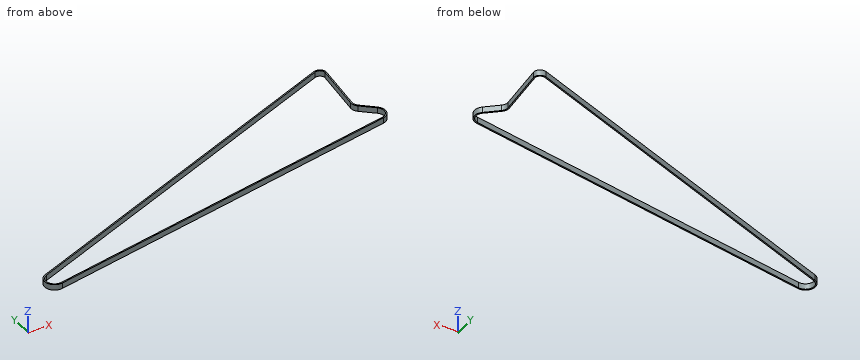
from build123d import *

# Parameters (mm, degrees)
SKETCH4_W = 6
SKETCH4_H = 1.45


with BuildPart() as part:
    # Sweep1: sweep along a path in Sketch2
    with BuildLine(Plane.XY) as sweep1_path:
        Line((6.634008087, 7.392396345), (-6.844115698, 19.487795186))
        ThreePointArc((-6.844115698, 19.487795186), (-9.188071123, 22.914875813), (-9.688379476, 27.036610909))
        Line((-9.688379476, 27.036610909), (-3.065681286, 82.544917251))
        ThreePointArc((-3.065681286, 82.544917251), (-5.437015562, 88.14522378), (-11.466030466, 88.943746635))
        Line((-11.466030466, 88.943746635), (-402.754294044, -70.804193152))
        ThreePointArc((-402.754294044, -70.804193152), (-408.510077554, -82.86635865), (-397.047352934, -89.738827246))
        Line((-397.047352934, -89.738827246), (1.95264707, -9.738827262))
        ThreePointArc((1.95264707, -9.738827262), (9.58135519, -2.618247459), (6.634008087, 7.392396345))
    # Sketch4 → Sweep1 (sweep)
    with BuildSketch(Plane(origin=(0, 0, 0), x_dir=(0, 0, 1), z_dir=(0.9804860480377625, 0.1965886812695244, 0))):
        with Locations((0, 9.932652567)):
            Rectangle(SKETCH4_W, SKETCH4_H)
    sweep(path=sweep1_path.line)


solid = part.part
Work out the finished part from the listing and answer in its coordinate system (mm). Coordinates: 2 decimals unless noted, no trailing zeros. Write each loop counter-clockwise with the first axis right and the second up, starting at its lowest first coordinate (ties: lowest second). Pieces come first, ordered by that corner, then holes.
1. The part is cut by section B-B, the plane y = 74. Write down the section's boundary in (x, z), and give its area (3 significant figures).
Results list:
outline: (-49.99, -3) - (-46.15, -3) - (-46.15, 3) - (-49.99, 3) - close; (-4.82, -3) - (-3.36, -3) - (-3.36, 3) - (-4.82, 3) - close
area: 31.8 mm2
2. Flat-ended cylindrical pins translate along their axes: pin 1 (3 mm diameter, centred on x = -115, z = -1.5, fed in from -Y); pin 2 (1.5 mm diameter, centred on y = -12, z = -2.5, fed in from -X); pin 3 (1 mm diameter, centred on y = 14.5, z = 0, fed in from +X). Find the tip coordinate at first contact, or state that the pin passes through.
Results list:
pin 1: stops at y = -34.23
pin 2: stops at x = -262.47
pin 3: stops at x = 0.36
3. The part is cut by section C-C, the plane x = -206. Write down the section's boundary in (y, z), and give its area (3 significant figures).
Results list:
outline: (-52.17, -3) - (-50.69, -3) - (-50.69, 3) - (-52.17, 3) - close; (8.74, -3) - (10.31, -3) - (10.31, 3) - (8.74, 3) - close
area: 18.3 mm2
4. Consider line 1 along X through (y, z) = (68, 0); line 2 along Y through (x, z) = (-119, 0); line 3 along Y through (x, z) = (-135.5, 1.9). Determine where each line is inside the solid, lowest interval first.
Results list:
line 1: x = -64.68 to -60.85, -5.53 to -4.07
line 2: y = -34.73 to -33.25, 44.26 to 45.82
line 3: y = -38.04 to -36.56, 37.52 to 39.09
